Work out the finished part from the listing and answer in its coordinate system (mm). Face numbers are marked on the shaded views. A direction names the side the tool comes from. Round coordinates to 2 decimals unless told otherwise and drop trailing zeros. Loops run counter-clockwise (first coordinate to the right, second up) from the corner with the lowest first, then second, coordinate; pieces in that order, holes last. Notation, with made-up numbers: (-35.75, 77) - (18.25, 77) arc R28 cw to (18.25, 111) - close; hole circle Ø3 at (53.25, -32.75). An arc over 180 degrees is marked (long way). Return JSON: item names as keys, results as strings.
from build123d import *

# Parameters (mm, degrees)
SKETCH1_R           = 41.275
SKETCH1_R_2         = 1.4732
SKETCH1_R_3         = 2
BOSS_EXTRUDE1_DEPTH = 6.0452
CUT_EXTRUDE3_DEPTH  = 59.683862288


with BuildPart() as part:
    # Sketch1 → Boss-Extrude1 (new body)
    with BuildSketch(Plane.XY):
        Circle(SKETCH1_R)
        with Locations((-6.35, 0)):
            Circle(SKETCH1_R_2, mode=Mode.SUBTRACT)
        with Locations((0, 6.35)):
            Circle(SKETCH1_R_2, mode=Mode.SUBTRACT)
        with Locations((6.35, 0)):
            Circle(SKETCH1_R_2, mode=Mode.SUBTRACT)
        with Locations((0, -6.35)):
            Circle(SKETCH1_R_2, mode=Mode.SUBTRACT)
        Circle(SKETCH1_R_3, mode=Mode.SUBTRACT)
    extrude(amount=BOSS_EXTRUDE1_DEPTH)

    # Sketch2 → Cut-Extrude3 (cut, through all)
    with BuildSketch(Plane.XY.offset(6.0452)):
        with BuildLine():
            Line((8.827105782, 17.78), (2.54, 25.272680903))
            ThreePointArc((2.54, 25.272680903), (15.758317518, 19.920728626), (24.009298775, 8.289365013))
            Line((24.009298775, 8.289365013), (14.484298775, 8.647939367))
            Line((14.484298775, 8.647939367), (9.404298775, 5.715))
            Line((9.404298775, 5.715), (12.637105782, 17.78))
            Line((12.637105782, 17.78), (8.827105782, 17.78))
        make_face()
        with BuildLine():
            Line((18.868143133, -3.140634987), (24.826209076, 5.368365013))
            ThreePointArc((24.826209076, 5.368365013), (20.911260009, -14.418016674), (3.81, -25.112624315))
            Line((3.81, -25.112624315), (3.81, -14.877877919))
            Line((3.81, -14.877877919), (16.51, -14.877877919))
            Line((16.51, -14.877877919), (11.327081569, -9.797877919))
            Line((11.327081569, -9.797877919), (21.487081569, -4.935568543))
            Line((21.487081569, -4.935568543), (18.868143133, -3.140634987))
        make_face()
        with BuildLine():
            Line((-3.81, -14.877877919), (-3.81, -25.112624315))
            ThreePointArc((-3.81, -25.112624315), (-20.911260009, -14.418016674), (-24.826209076, 5.368365013))
            Line((-24.826209076, 5.368365013), (-18.868143133, -3.140634987))
            Line((-18.868143133, -3.140634987), (-21.487081569, -4.935568543))
            Line((-21.487081569, -4.935568543), (-11.327081569, -9.797877919))
            Line((-11.327081569, -9.797877919), (-16.51, -14.877877919))
            Line((-16.51, -14.877877919), (-3.81, -14.877877919))
        make_face()
        with BuildLine():
            Line((-14.484298775, 8.647939367), (-24.009298775, 8.289365013))
            ThreePointArc((-24.009298775, 8.289365013), (-15.758317518, 19.920728626), (-2.54, 25.272680903))
            Line((-2.54, 25.272680903), (-8.827105782, 17.78))
            Line((-8.827105782, 17.78), (-12.637105782, 17.78))
            Line((-12.637105782, 17.78), (-9.404298775, 5.715))
            Line((-9.404298775, 5.715), (-14.484298775, 8.647939367))
        make_face()
    extrude(amount=-CUT_EXTRUDE3_DEPTH, mode=Mode.SUBTRACT)


solid = part.part
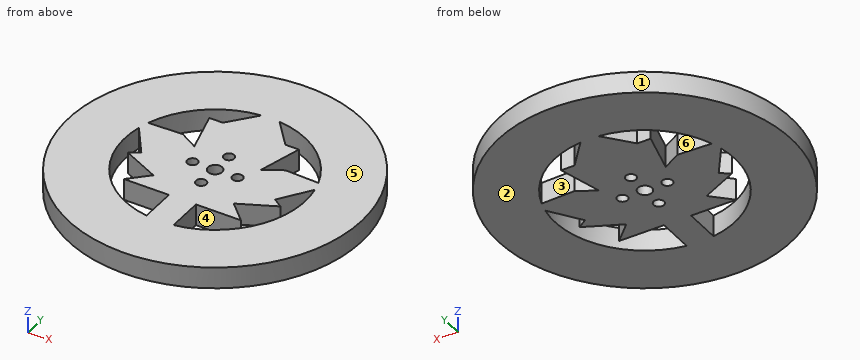
1) Find the intervals of material crossed by L1, parallel to Y at x = 0, z = 3 (3 decimals); L2, parallel to X at y = 22, z = 4; L3, parallel to X at y = 0.5, z = 1.75, in increasing order.
Verdict:
{"L1": "y = -41.275 to -7.823, -4.877 to -2, 2 to 4.877, 7.823 to 41.275", "L2": "x = -34.92 to -12.69, -5.29 to 5.29, 12.69 to 34.92", "L3": "x = -41.27 to -25.4, -21.42 to -7.74, -4.96 to -1.94, 1.94 to 4.96, 7.74 to 21.42, 25.4 to 41.27"}
2) Flat-ended cylindrical pins translate along their axes: pin 1 (2.5 mm diameter, centred on x = -6.35, y = 0, fed in from -Z); pin 2 (3 mm diameter, centred on x = -9, z = 1.5, fed in from -Y); pin 3 (2 mm diameter, centred on x = -13, z = 1.5, fed in from -Y); pin 4 (2 mm diameter, centred on x = 27, z = 5, fed in from -Y). Find the tip coordinate at first contact, or state that the pin passes through.
Verdict:
{"pin 1": "passes through", "pin 2": "stops at y = -40.59", "pin 3": "stops at y = -39.49", "pin 4": "stops at y = -32.06"}
3) Section A-A (z = 3) is taken. Count the separate pieces of the cut face and the enclosed holes in it, and give its area (3 significant figures).
Verdict:
{"separate pieces": "1", "enclosed holes": "9", "area": "4,550 mm2"}
4) A tool of negligible diameter and unlimited length cuts with its end or side. For the marked faces 5 and 6, from which of +Z, -Z, +X, -X, +Y, -Y can it reach the whole face along a straight path? Write none if from no direction.
Verdict:
{"face 5": "+Z, +X, -X, +Y, -Y", "face 6": "+Z, -Z"}
5) Section B-B (x = 0) is taken. Give the vertices of the cut face in (y, z) (3 decimals), and give its area (3 significant figures).
Verdict:
{"outline": "(-41.275, 0) - (-7.823, 0) - (-7.823, 6.045) - (-41.275, 6.045) - close; (-4.877, 0) - (-2, 0) - (-2, 6.045) - (-4.877, 6.045) - close; (2, 0) - (4.877, 0) - (4.877, 6.045) - (2, 6.045) - close; (7.823, 0) - (41.275, 0) - (41.275, 6.045) - (7.823, 6.045) - close", "area": "439 mm2"}
6) Section D-D (y = 22) is taken. Give the vertices of the cut face in (x, z), and give its area (3 significant figures).
Verdict:
{"outline": "(-34.92, 0) - (-12.69, 0) - (-12.69, 6.05) - (-34.92, 6.05) - close; (-5.29, 0) - (5.29, 0) - (5.29, 6.05) - (-5.29, 6.05) - close; (12.69, 0) - (34.92, 0) - (34.92, 6.05) - (12.69, 6.05) - close", "area": "333 mm2"}
7) Determine the mould class of the marked faces 1, 2, 3 and 4 for opening direction Y: pulls with the +Y half, pulls with the -Y half, needs draft (parallel to the pull), parting line crosses it, or undercut.
Verdict:
{"face 1": "parting line crosses it", "face 2": "needs draft", "face 3": "undercut", "face 4": "undercut"}
8) Section C-C (y = 0) is taken. Give the vertices of the cut face in (x, z) (3 decimals).
Verdict:
{"outline": "(-41.275, 0) - (-25.4, 0) - (-25.4, 6.045) - (-41.275, 6.045) - close; (-21.067, 0) - (-7.823, 0) - (-7.823, 6.045) - (-21.067, 6.045) - close; (-4.877, 0) - (-2, 0) - (-2, 6.045) - (-4.877, 6.045) - close; (2, 0) - (4.877, 0) - (4.877, 6.045) - (2, 6.045) - close; (7.823, 0) - (21.067, 0) - (21.067, 6.045) - (7.823, 6.045) - close; (25.4, 0) - (41.275, 0) - (41.275, 6.045) - (25.4, 6.045) - close"}
